Check sheet for the drawn part. Datum: minimum x, y, z corner. Units: mm. A direction names the side the tool comes from. Give positions to 0.01 mm unless a question says otherwise; leave off trailing zeros. Write each loop counter-clockwise with the first axis right and the second up, starting at its lowest first coordinate (ties: lowest second). Pieces come first, ordered by that corner, then holes. Notation, with made-up numbers: M -35,17.25 L -12,17.25 A10 ccw -12,31.25 Z; hole C 70.5,70 d1. An arc over 180 degrees is marked long. Use CSV: the item, a comma, the result in double quotes. Start each with the question number.
1. Access from +Z, -Z, +X, -X, +Y, -Y to the whole of each face (thin tool, end or side, straight path). Record for the marked faces 1 and 2.
2. Scan lines: line 1 (X direction, y = 58.5, z = 43.5); line 2 (Y direction, x = 43.5, z = 49.5); line 3 (Y direction, x = 90.5, z = 36.5). Record each from-to range of solid material in increasing order.
3. Cross-section at C-C, the plane x = 64. Enter the section's corners in (y, z).
4. Cross-section at D-D, the plane y = 12.5. Enter the section's corners in (x, z).
5. Cross-section at A-A, the plane z = 36. Enter the section's corners in (x, y).
6. Depth check by flat-ended pin: P1, Ø2, axis at x = 95.5, z = 24.5, coming from the +Y side; P2, Ø4, axis at x = 16.5, y = 47, coming from the +Z side; P3, Ø8, axis at y = 64, z = 9.5, coming from the -X side. Enter the tip coordinate at first touch or a pass-through.
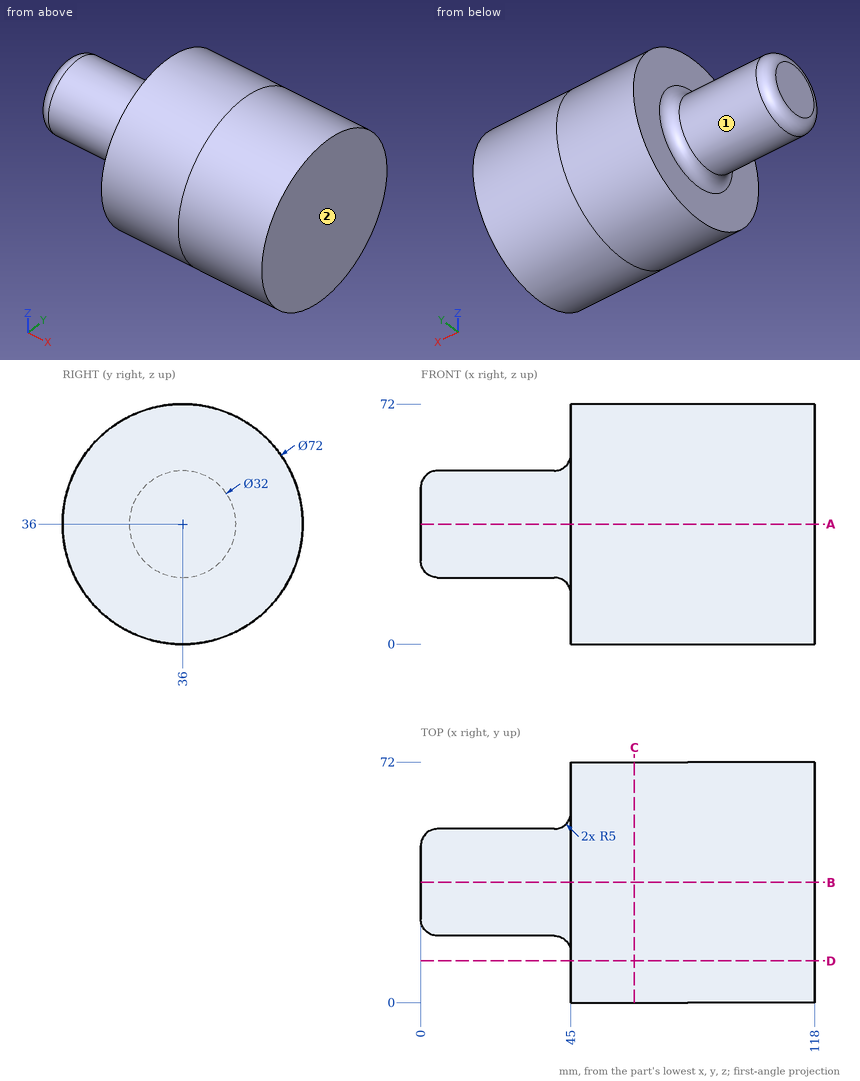
Worked answers:
1,face 1,"-X"
1,face 2,"+Z, -Z, +X, +Y, -Y"
2,line 1,"x = 45 to 118"
2,line 2,"y = 24.98 to 47.02"
2,line 3,"y = 0 to 72"
3,outline,"C 36,36 d72"
4,outline,"M 45,8.73 L 118,8.73 L 118,63.27 L 45,63.27 Z"
5,outline,"M 0,25 A5 ccw 5,20 L 40,20 A5 cw 45,15 L 45,0 L 118,0 L 118,72 L 45,72 L 45,57 A5 cw 40,52 L 5,52 A5 ccw 0,47 Z"
6,P1,"stops at y = 70.43"
6,P2,"stops at z = 49.23"
6,P3,"stops at x = 45"
